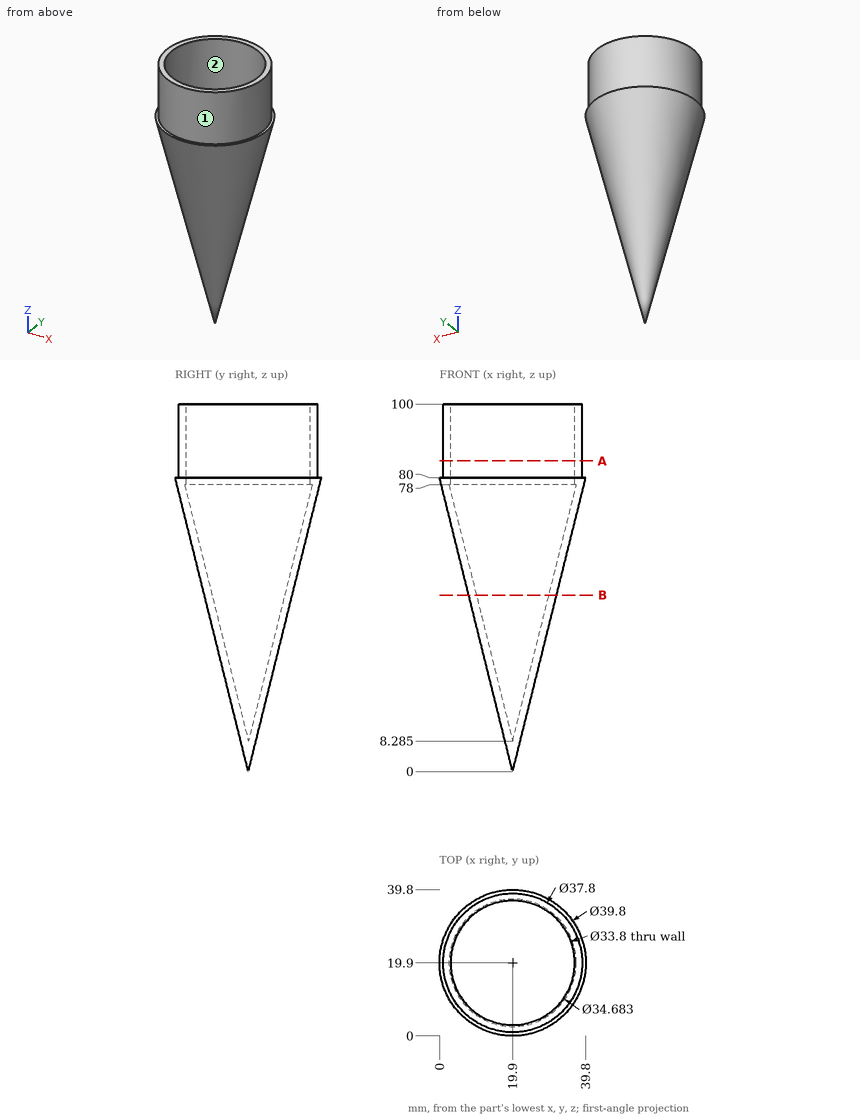
Study the drawing (mm; zero at the part's minimum x, y, z) and answer. Give positions to 0.01 mm unless a question says otherwise; leave off trailing zeros. Write each loop counter-clockwise with the first axis right and the second up, starting at its lowest first coordinate (ties: lowest second). Pieces come first, ordered by that corner, then holes.
Item 1: Find the intervals of material crossed by line 1 along Y through (x, z) = (19.9, 86.75); line 2 along X through (y, z) = (30, 69.5) (1 decimal); line 3 along X through (y, z) = (19, 90), in increasing order.
Item 2: Determine the mould class of the marked faces 1 and 2 for opening direction Y: released by +Y, released by -Y, zero draft, split by the parting line, or undercut.
Item 3: Section B-B, the plane z = 48 is taken. Write down the section's boundary in (x, y), plus the area to 3 significant figures.
Item 4: Flat-ended cylindrical pins translate along their axes: P1, Ø20, axis at x = 29, y = 25.5, coming from the +Z side; P2, Ø3, axis at x = 16.5, z = 51.5, coming from the -Y side; P3, Ø6, axis at x = 18, z = 16, coming from the +Y side. Find the tip coordinate at first contact, or state that the pin passes through.
Item 5: Section A-A, the plane z = 84.5 is taken. Write down the section's boundary in (x, y).
Completed:
1. line 1: y = 1 to 3, 36.8 to 38.8
1. line 2: x = 5.9 to 8.5, 31.3 to 33.9
1. line 3: x = 1.02 to 3.02, 36.78 to 38.78
2. face 1: split by the parting line
2. face 2: undercut
3. outline: circle Ø23.88 at (19.9, 19.9); hole circle Ø19.76 at (19.9, 19.9)
3. area: 141 mm2
4. P1: stops at z = 100
4. P2: stops at y = 7.03
4. P3: stops at y = 24.51
5. outline: circle Ø37.8 at (19.9, 19.9); hole circle Ø33.8 at (19.9, 19.9)
